from build123d import *

# Parameters (mm, degrees)
CROQUIS1_R                = 22.5
CROQUIS1_R_2              = 20.9
SALIENTE_EXTRUIR1_DEPTH   = 30
CROQUIS1_R_3              = 29.95
CROQUIS1_R_4              = 28.75
SALIENTE_EXTRUIR1_2_DEPTH = 30
CORTAR_EXTRUIR1_DEPTH     = 30
SALIENTE_EXTRUIR2_DEPTH   = 4


with BuildPart() as part:
    # Croquis1 → Saliente-Extruir1 (new body)
    with BuildSketch(Plane.XY):
        Circle(CROQUIS1_R)
        Circle(CROQUIS1_R_2, mode=Mode.SUBTRACT)
    extrude(amount=SALIENTE_EXTRUIR1_DEPTH)

    # Croquis2 → Cortar-Extruir1 (cut)
    with BuildSketch(Plane.XY.offset(30)):
        with BuildLine():
            ThreePointArc((3.907083998, 22.158174443), (1.961004212, 22.414380707), (0, 22.5))
            Line((0, 22.5), (0, 21.999786926))
            ThreePointArc((0, 21.999786926), (1.91740777, 21.916071095), (3.820222909, 21.66556073))
            Line((3.820222909, 21.66556073), (3.907083998, 22.158174443))
        make_face()
        with BuildLine():
            ThreePointArc((-3.820222909, -21.66556073), (-1.91740777, -21.916071095), (0, -21.999786926))
            Line((0, -21.999786926), (0, -22.5))
            ThreePointArc((0, -22.5), (-1.961004212, -22.414380707), (-3.907083998, -22.158174443))
            Line((-3.907083998, -22.158174443), (-3.820222909, -21.66556073))
        make_face()
        with BuildLine():
            ThreePointArc((-22.158174443, 3.907083998), (-22.414380707, 1.961004212), (-22.5, 0))
            Line((-22.5, 0), (-21.999786926, 0))
            ThreePointArc((-21.999786926, 0), (-21.916071095, 1.91740777), (-21.66556073, 3.820222909))
            Line((-21.66556073, 3.820222909), (-22.158174443, 3.907083998))
        make_face()
    extrude(amount=-CORTAR_EXTRUIR1_DEPTH, mode=Mode.SUBTRACT)



with BuildPart() as body_2:
    # Croquis1 → Saliente-Extruir1 2 (new body)
    with BuildSketch(Plane.XY):
        Circle(CROQUIS1_R_3)
        Circle(CROQUIS1_R_4, mode=Mode.SUBTRACT)
    extrude(amount=SALIENTE_EXTRUIR1_2_DEPTH)


with BuildPart() as part_1:
    add(part.part)

    add(body_2.part)  # Saliente-Extruir2 merges body 2
    # Croquis3 → Saliente-Extruir2 (add)
    with BuildSketch(Plane(origin=(0, 0, 0), x_dir=(-1, 0, 0), z_dir=(0, 0, -1))):
        with BuildLine():
            ThreePointArc((-18.484895437, 12.828041187), (-15.909902577, 15.909902577), (-12.828041187, 18.484895437))
            Line((-12.828041187, 18.484895437), (-18.159694516, 23.816548765))
            Line((-18.159694516, 23.816548765), (-23.816548765, 18.159694516))
            Line((-23.816548765, 18.159694516), (-18.484895437, 12.828041187))
        make_face()
        with BuildLine():
            Line((-18.159694516, -23.816548765), (-12.828041187, -18.484895437))
            ThreePointArc((-12.828041187, -18.484895437), (-15.909902577, -15.909902577), (-18.484895437, -12.828041187))
            Line((-18.484895437, -12.828041187), (-23.816548765, -18.159694516))
            Line((-23.816548765, -18.159694516), (-18.159694516, -23.816548765))
        make_face()
        with BuildLine():
            Line((23.816548765, -18.159694516), (18.484895437, -12.828041187))
            ThreePointArc((18.484895437, -12.828041187), (15.909902577, -15.909902577), (12.828041187, -18.484895437))
            Line((12.828041187, -18.484895437), (18.159694516, -23.816548765))
            Line((18.159694516, -23.816548765), (23.816548765, -18.159694516))
        make_face()
        with BuildLine():
            Line((18.484895437, 12.828041187), (23.816548765, 18.159694516))
            Line((23.816548765, 18.159694516), (18.159694516, 23.816548765))
            Line((18.159694516, 23.816548765), (12.828041187, 18.484895437))
            ThreePointArc((12.828041187, 18.484895437), (15.909902577, 15.909902577), (18.484895437, 12.828041187))
        make_face()
    extrude(amount=-SALIENTE_EXTRUIR2_DEPTH)


solid = part_1.part
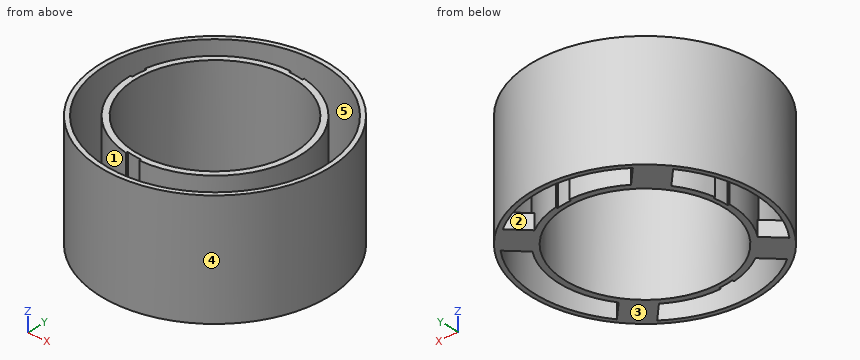
Build history of the part. All positions in model axes, mm. Face numbers are marked on the shaded views. A direction names the side the tool comes from. Give positions to 0.01 mm unless a question says otherwise; leave off trailing zeros. Order: outer loops, then holes, each group sorted by start corner. A loop starts at its lowest first (then second) coordinate and runs counter-clockwise, first axis right, second up. Notation, with made-up numbers: M -16,58.5 L 23,58.5 A32 ccw 23,84.5 Z; hole C 76.5,25 d10. An arc over 180 degrees is marked long. Put each result on its own line as item: value.
Item 1: Slice it at B-B, the plane x = -5. Write the cut outline in (y, z).
From the geometry:
outline: M -29.53,0 L -28.31,0 L -28.31,30 L -29.53,30 Z; M -21.94,0 L -20.29,0 L -20.29,30 L -21.94,30 Z; M 20.29,0 L 21.94,0 L 21.94,30 L 20.29,30 Z; M 28.31,0 L 29.53,0 L 29.53,30 L 28.31,30 Z
Item 2: Slice it at C-C, the plane y = -20. Write the cut outline in (x, z), plus the area to 3 significant figures.
From the geometry:
outline: M -22.29,0 L -14.34,0 L -14.34,4 L -20.65,4 L -20.65,30 L -22.29,30 Z; M -10.31,0 L -6.07,0 L -6.07,30 L -10.31,30 Z; M 6.07,0 L 10.31,0 L 10.31,30 L 6.07,30 Z; M 14.34,0 L 22.29,0 L 22.29,30 L 20.65,30 L 20.65,4 L 14.34,4 Z
area: 403 mm2
Item 3: 3-axis set-ups, long thin cutter, end or side, ignore diameter. For the marked faces 1 and 2: which of +Z, -Z, +X, -X, +Y, -Y reach the whole face in a straight line?
From the geometry:
face 1: +Z
face 2: +Z, -Z
Item 4: Two-plate mould, pull along X, no slides. Class the marked faces 3, 4 and 5: +X half, -X half, draft (parallel to the pull), parting line (faces both ways), or undercut.
From the geometry:
face 3: draft
face 4: parting line
face 5: undercut
Item 5: Slice it at A-A, the plane z = 22.5. Write the cut outline in (x, y).
From the geometry:
outline: C 0,0 d59.9; M -22.5,0 A22.5 ccw -3.91,-22.16 L -3.82,-21.67 A22 ccw 0,-22 L 0,-22.5 A22.5 ccw 3.91,22.16 L 3.82,21.67 A22 ccw 0,22 L 0,22.5 A22.5 ccw -22.16,3.91 L -21.67,3.82 A22 ccw -22,0 Z; hole C 0,0 d57.5; hole C 0,0 d41.8
Item 6: Probe line 1 (Y direction, x = 2.5, z = 27.75); line 2 (Y direction, x = -12.5, z = 19.75); line 3 (X direction, y = -4.5, z = 2.25). List the from-to ranges inside material, lowest first. Write a range as [from, to].
From the geometry:
line 1: y = [-29.85, -28.64], [-22.36, -20.75], [20.75, 21.86], [28.64, 29.85]
line 2: y = [-27.22, -25.89], [-18.71, -16.75], [16.75, 18.71], [25.89, 27.22]
line 3: x = [-29.61, -28.4], [-22.05, -20.41], [20.41, 22.05], [28.4, 29.61]
Item 7: Slice it at D-D, the plane y = 16. Write the cut outline in (x, z).
From the geometry:
outline: M -25.32,0 L -23.89,0 L -23.89,30 L -25.32,30 Z; M -21.66,0 L -13.45,0 L -13.45,30 L -15.82,30 L -15.82,4 L -21.66,4 Z; M 13.45,0 L 21.66,0 L 21.66,4 L 15.82,4 L 15.82,30 L 13.45,30 Z; M 23.89,0 L 25.32,0 L 25.32,30 L 23.89,30 Z
Item 8: Flat gauge pins, fed straight in: pin 1 Ø6 at (x, z) = (18, 14) entering from -Y; pin 2 Ø8 at (x, z) = (-20.5, 18.5) entering from +Y; pin 3 Ø4 at (x, z) = (9.5, 12) entering from -Y. Where does each tip first touch, or does it go through?
From the geometry:
pin 1: stops at y = -25.92
pin 2: stops at y = 25
pin 3: stops at y = -29
